Read the model definition and answer for the solid it produces. Units are mm, in the model's axes. A direction names the side the tool comes from. Round coordinates to 2 decimals unless told otherwise and drop trailing zeros. Loops run counter-clockwise (first coordinate to the right, second up) from the corner with the lowest first, then second, coordinate; pieces in that order, holes last. Notation, with made-up numbers: (-22, 83.25) - (24, 83.25) arc R20 cw to (24, 88.25) - close; hole circle Ø10 at (-28.5, 38). An arc over 180 degrees is marked (long way). Answer as CSV lines item,"result".
```python
from build123d import *

# Parameters (mm, degrees)
BOSS_EXTRUDE1_DEPTH = 10
CUT_EXTRUDE1_REACH  = 15.4
SKETCH2_R           = 2.25
SKETCH2_R_2         = 1.6
CUT_EXTRUDE2_DEPTH  = 7.4
CUT_EXTRUDE3_DEPTH  = 7.4


with BuildPart() as part:
    # Sketch1 → Boss-Extrude1 (new body, symmetric)
    with BuildSketch(Plane.XY):
        with BuildLine():
            Line((17.453939383, -30.6), (-17.453939383, -30.6))
            ThreePointArc((-17.453939383, -30.6), (-20.972536151, -33.54882923), (-24, -37))
            Line((-24, -37), (-24, -44))
            Line((-24, -44), (24, -44))
            Line((24, -44), (24, -37))
            ThreePointArc((24, -37), (20.972536151, -33.54882923), (17.453939383, -30.6))
        make_face()
    extrude(amount=BOSS_EXTRUDE1_DEPTH, both=True)

    # Sketch2 → Cut-Extrude1 (cut, up to next)
    with BuildSketch(Plane(origin=(0, -30.6, 0), x_dir=(1, 0, 0), z_dir=(0, 1, 0)), mode=Mode.PRIVATE) as cut_extrude1_sk1:
        Circle(SKETCH2_R)
    cut_extrude1_tool1 = extrude(cut_extrude1_sk1.sketch, amount=-CUT_EXTRUDE1_REACH, mode=Mode.PRIVATE) & part.part
    add(cut_extrude1_tool1.solids().sort_by_distance((0, -30.6, 0))[0], mode=Mode.SUBTRACT)
    # Sketch2 → Cut-Extrude1 (cut, up to next)
    with BuildSketch(Plane(origin=(0, -30.6, 0), x_dir=(1, 0, 0), z_dir=(0, 1, 0)), mode=Mode.PRIVATE) as cut_extrude1_sk2:
        with Locations((-10, 0)):
            Circle(SKETCH2_R_2)
    cut_extrude1_tool2 = extrude(cut_extrude1_sk2.sketch, amount=-CUT_EXTRUDE1_REACH, mode=Mode.PRIVATE) & part.part
    add(cut_extrude1_tool2.solids().sort_by_distance((-10, -30.6, 0))[0], mode=Mode.SUBTRACT)
    # Sketch2 → Cut-Extrude1 (cut, up to next)
    with BuildSketch(Plane(origin=(0, -30.6, 0), x_dir=(1, 0, 0), z_dir=(0, 1, 0)), mode=Mode.PRIVATE) as cut_extrude1_sk3:
        with Locations((10, 0)):
            Circle(SKETCH2_R_2)
    cut_extrude1_tool3 = extrude(cut_extrude1_sk3.sketch, amount=-CUT_EXTRUDE1_REACH, mode=Mode.PRIVATE) & part.part
    add(cut_extrude1_tool3.solids().sort_by_distance((10, -30.6, 0))[0], mode=Mode.SUBTRACT)

    # Sketch3 → Cut-Extrude2 (cut)
    with BuildSketch(Plane(origin=(0, -30.6, 0), x_dir=(1, 0, 0), z_dir=(0, 1, 0))):
        Polygon((-10, -3.233161507), (-7.2, -1.616580754), (-7.2, 1.616580754), (-10, 3.233161507), (-12.8, 1.616580754), (-12.8, -1.616580754), align=None)
        Polygon((10, -3.233161507), (7.2, -1.616580754), (7.2, 1.616580754), (10, 3.233161507), (12.8, 1.616580754), (12.8, -1.616580754), align=None)
    extrude(amount=-CUT_EXTRUDE2_DEPTH, mode=Mode.SUBTRACT)

    # Sketch4 → Cut-Extrude3 (cut)
    with BuildSketch(Plane.XZ.offset(44)):
        Polygon((0, -4.041451884), (3.5, -2.020725942), (3.5, 2.020725942), (0, 4.041451884), (-3.5, 2.020725942), (-3.5, -2.020725942), align=None)
    extrude(amount=-CUT_EXTRUDE3_DEPTH, mode=Mode.SUBTRACT)


solid = part.part
```
1) A cutting plane is placed at B-B, the plane z = -7. Determine the outline of the cut face in (x, y).
Entries:
outline,"(-24, -44) - (24, -44) - (24, -37) arc R30 ccw to (17.45, -30.6) - (-17.45, -30.6) arc R30 ccw to (-24, -37) - close"
2) A cutting plane is placed at A-A, the plane y = -42.5. Determine the outline of the cut face in (x, z).
Entries:
outline,"(-24, -10) - (24, -10) - (24, 10) - (-24, 10) - close; hole circle Ø3.2 at (-10, 0); hole (-3.5, -2.02) - (0, -4.04) - (3.5, -2.02) - (3.5, 2.02) - (0, 4.04) - (-3.5, 2.02) - close; hole circle Ø3.2 at (10, 0)"
3) A tool of negligible diameter and unlimited length cuts with its end or side. For faces 5 (the face through (8.62, -34.248, 2.436)), 6 (the face through (-1.726, -40.352, 3.045)), 7 (the face through (0, -37, -10)), from which of +Z, -Z, +X, -X, +Y, -Y can it reach the whole face along a straight path? Write none if from no direction.
Entries:
face 5,"+Y"
face 6,"-Y"
face 7,"-Z, +X, -X, +Y, -Y"
4) Find the intervals of material crossed by line 1 (X direction, y = -42.2, z = 0); line 2 (Z direction, x = 10, y = -41); line 3 (X direction, y = -33.2, z = 0), in increasing order.
Entries:
line 1,"x = -24 to -11.6, -8.4 to -3.5, 3.5 to 8.4, 11.6 to 24"
line 2,"z = -10 to -1.6, 1.6 to 10"
line 3,"x = -20.61 to -12.8, -7.2 to -2.25, 2.25 to 7.2, 12.8 to 20.61"
5) A cutting plane is placed at D-D, the plane y = -32. Determine the outline of the cut face in (x, z).
Entries:
outline,"(-19.26, -10) - (19.26, -10) - (19.26, 10) - (-19.26, 10) - close; hole (-12.8, -1.62) - (-10, -3.23) - (-7.2, -1.62) - (-7.2, 1.62) - (-10, 3.23) - (-12.8, 1.62) - close; hole circle Ø4.5 at (0, 0); hole (7.2, -1.62) - (10, -3.23) - (12.8, -1.62) - (12.8, 1.62) - (10, 3.23) - (7.2, 1.62) - close"
6) Each of these flat-tipped pins is pushed along its axis until it touches: P1, Ø5, axis at x = 0, z = 0, coming from the -Y side; P2, Ø1.7, axis at x = -9.5, z = 1.5, coming from the +Y side; P3, Ø1.6, axis at y = -34, z = 0.5, coming from the +X side; P4, Ø1.9, axis at x = 10, z = 0, coming from the -Y side. Where does it stop, or does it pass through?
Entries:
P1,"stops at y = -36.6"
P2,"stops at y = -38"
P3,"stops at x = 22.18"
P4,"passes through"
7) The mould has two halves that part along X. Classify faces 1 (the face through (21.018, -33.594, 0.14)), 2 (the face through (-24, -40, 0)), 3 (the face through (-11.42, -34.248, 2.414)), 4 (the face through (-8.62, -34.248, 2.436)): pulls with the +X half, pulls with the -X half, needs draft (parallel to the pull), parting line crosses it, or undercut.
Entries:
face 1,"pulls with the +X half"
face 2,"pulls with the -X half"
face 3,"undercut"
face 4,"undercut"
8) A cutting plane is placed at C-C, the plane y = -35.5. Determine the outline of the cut face in (x, z).
Entries:
outline,"(-22.8, -10) - (22.8, -10) - (22.8, 10) - (-22.8, 10) - close; hole (-12.8, -1.62) - (-10, -3.23) - (-7.2, -1.62) - (-7.2, 1.62) - (-10, 3.23) - (-12.8, 1.62) - close; hole circle Ø4.5 at (0, 0); hole (7.2, -1.62) - (10, -3.23) - (12.8, -1.62) - (12.8, 1.62) - (10, 3.23) - (7.2, 1.62) - close"
